from build123d import *

# Parameters (mm, degrees)
SKETCH1_R           = 4
BOSS_EXTRUDE1_DEPTH = 5
SKETCH2_R           = 5.2
BOSS_EXTRUDE2_DEPTH = 2
SKETCH3_R           = 1.25
CUT_EXTRUDE2_DEPTH  = 8
CHAMFER1_SIZE       = 0.4
SKETCH4_W           = 20
SKETCH4_H           = 0.8
CUT_EXTRUDE3_DEPTH  = 1.4
SKETCH5_R           = 2
CUT_EXTRUDE4_DEPTH  = 2.5
FILLET1_R           = 0.5


with BuildPart() as part:
    # Sketch1 → Boss-Extrude1 (new body)
    with BuildSketch(Plane.XY):
        with Locations((1.5, 95.99791663)):
            Circle(SKETCH1_R)
    extrude(amount=BOSS_EXTRUDE1_DEPTH)

    # Sketch2 → Boss-Extrude2 (add)
    with BuildSketch(Plane(origin=(0, 0, 0), x_dir=(-1, 0, 0), z_dir=(0, 0, -1))):
        with Locations((-1.5, 95.99791663)):
            Circle(SKETCH2_R)
    extrude(amount=BOSS_EXTRUDE2_DEPTH)

    # Sketch3 → Cut-Extrude2 (cut, through all)
    with BuildSketch(Plane.XY.offset(5)):
        with Locations((0, 95.99791663)):
            Circle(SKETCH3_R)
    extrude(amount=-CUT_EXTRUDE2_DEPTH, mode=Mode.SUBTRACT)

    # Chamfer1
    chamfer1_edges = [part.edges().sort_by_distance(p)[0] for p in [
        (-2.5, 95.99791663, 5),
        (6.7, 95.99791663, -2),
    ]]
    chamfer(chamfer1_edges, length=CHAMFER1_SIZE)

    # Sketch4 → Cut-Extrude3 (cut)
    with BuildSketch(Plane(origin=(0, 0, -2), x_dir=(-1, 0, 0), z_dir=(0, 0, -1))):
        with Locations((-1.5, 95.99791663)):
            Rectangle(SKETCH4_W, SKETCH4_H)
    extrude(amount=-CUT_EXTRUDE3_DEPTH, mode=Mode.SUBTRACT)

    # Sketch5 → Cut-Extrude4 (cut)
    with BuildSketch(Plane(origin=(0, 0, -2), x_dir=(-1, 0, 0), z_dir=(0, 0, -1))):
        with Locations((0, 95.99791663)):
            Circle(SKETCH5_R)
    extrude(amount=-CUT_EXTRUDE4_DEPTH, mode=Mode.SUBTRACT)

    # Fillet1
    fillet1_edges = [part.edges().sort_by_distance(p)[0] for p in [
        (2, 95.99791663, 0.5),
    ]]
    fillet(fillet1_edges, radius=FILLET1_R)


solid = part.part
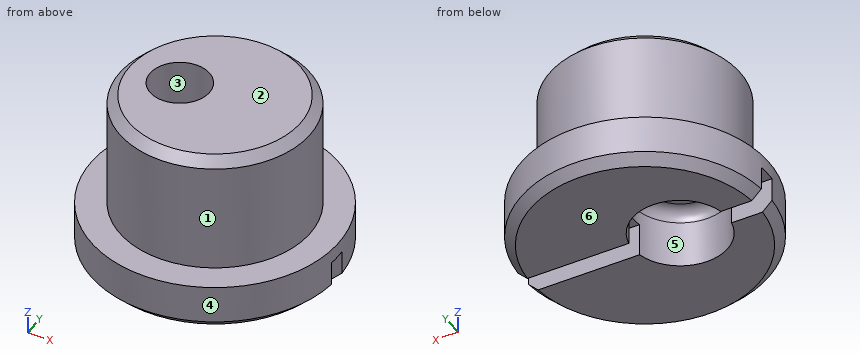
Input: part model. Units: mm. Frame: model coordinates. Face numbers are marked on the shaded views. A direction names the side the tool comes from. Coordinates: 2 decimals unless noted, no trailing zeros. Loops run counter-clockwise (first coordinate to the right, second up) from the corner with the lowest first, then second, coordinate; pieces in that order, holes last.
(1) Section A-A on z = 1. Return the cut outline in (x, y), then the cut area to 3 significant figures.
(2) Set-up query: the marked faces 1 and 2. Return all of +Z, -Z, +X, -X, +Y, -Y with unobstructed straight access to the full face (end or side cutting, diameter ignored); none if empty.
(3) Material intervals for probe 1 along Y at (x, z) = (0, -1); probe 2 along X at (y, z) = (97.75, -0.25); probe 3 along X at (y, z) = (95, -1), sorted ascending.
(4) Pull-direction query (X, two-part tool) for the marked faces 3, 4, 5 and 6; classes: released by +X, released by -X, zero draft, split by the parting line, or undercut.
(5) First-contact query: pin 1 Ø1.1 at (x, z) = (-2.5, -1) entering from -Y; pin 2 Ø1.5 at (x, z) = (4.5, -1.5) entering from +Y; pin 3 Ø0.7 at (x, z) = (-2.5, -1) entering from +Y. Flat tips, straight axial feed; report the tip coordinate or a pass-through.
Data:
1. outline: circle Ø8 at (1.5, 96); hole circle Ø2.5 at (0, 96)
1. area: 45.4 mm2
2. face 1: +Z
2. face 2: +Z, +X, -X, +Y, -Y
3. probe 1: y = 91.02 to 94, 98 to 100.98
3. probe 2: x = -3.4 to -0.96, 0.96 to 6.4
3. probe 3: x = -3.6 to -1.73, 1.73 to 6.6
4. face 3: undercut
4. face 4: split by the parting line
4. face 5: undercut
4. face 6: zero draft
5. pin 1: stops at y = 92.11
5. pin 2: stops at y = 100.69
5. pin 3: stops at y = 99.7
